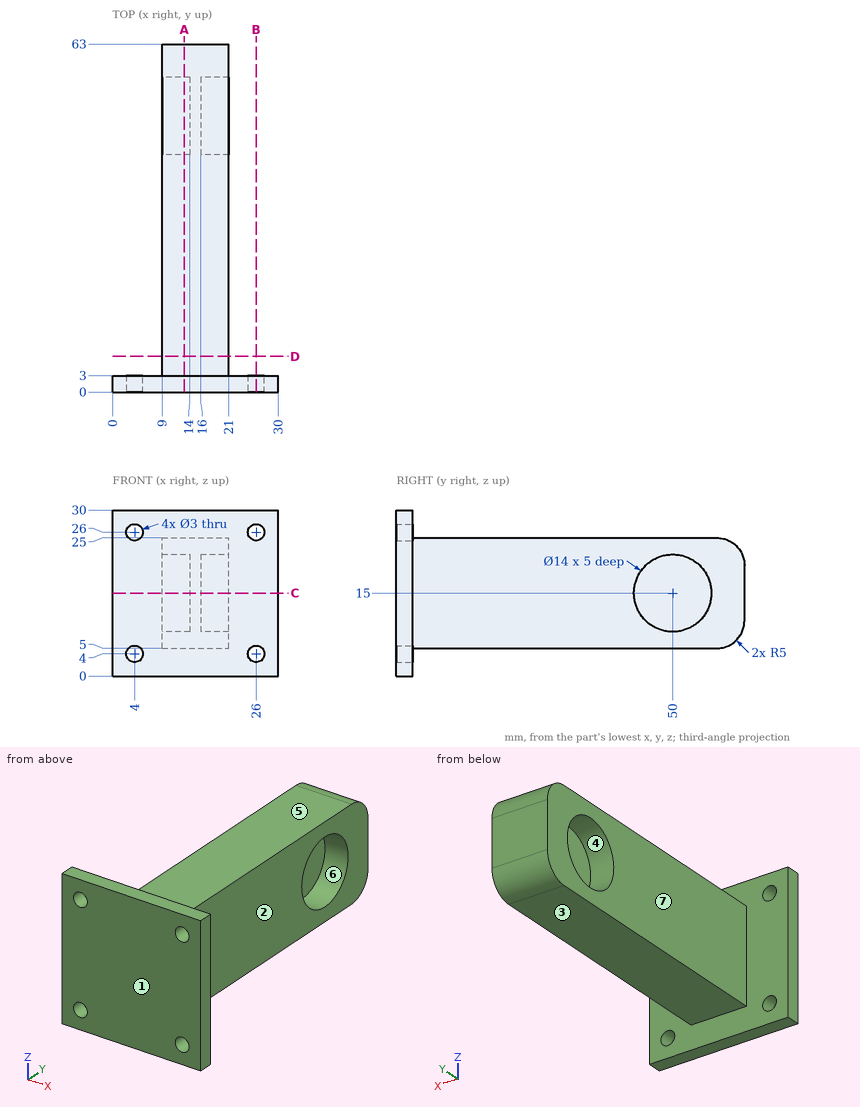
Job drawing, mm, ordinate dimensions from the low corner. One solid piece. A direction names the side the tool comes from. Give positions to 0.01 mm unless a question says otherwise; leave off trailing zeros. Write each loop counter-clockwise with the first axis right and the second up, starting at its lowest first coordinate (ties: lowest second). Pieces come first, ordered by that corner, then holes. Notation, with made-up numbers: (59, 70.25) - (92, 70.25) arc R22 cw to (92, 85.25) - close; hole circle Ø11 at (3.25, 75.25). An arc over 180 degrees is marked (long way). Answer as CSV lines item,"result".
1. Band-saw the part on C-C (z = 15). Write the cut outline in (x, y), and give its area (3 significant figures).
Responses:
outline,"(0, 0) - (30, 0) - (30, 3) - (21, 3) - (21, 43) - (16, 43) - (16, 57) - (21, 57) - (21, 63) - (9, 63) - (9, 57) - (14, 57) - (14, 43) - (9, 43) - (9, 3) - (0, 3) - close"
area,"670 mm2"
2. Pin check, flat tips, straight feed: pin 1 (18 mm diameter, centred on y = 50, z = 15, fed in from +X); pin 2 (3 mm diameter, centred on x = 19.5, y = 48.5, fed in from +Z); pin 3 (10 mm diameter, centred on y = 26, z = 14.5, fed in from -X); pin 4 (12 mm diameter, centred on x = 23, z = 13, fed in from +Y). Stop position of each tip, or through.
Responses:
pin 1,"stops at x = 21"
pin 2,"stops at z = 25"
pin 3,"stops at x = 9"
pin 4,"stops at y = 63"
3. Band-saw the part on A-A (x = 13). Write the cut outline in (y, z).
Responses:
outline,"(0, 0) - (3, 0) - (3, 5) - (58, 5) arc R5 ccw to (63, 10) - (63, 20) arc R5 ccw to (58, 25) - (3, 25) - (3, 30) - (0, 30) - close; hole circle Ø14 at (50, 15)"
4. Two-plate mould, pull along Z, no slides. Class the marked faces 4, 5, 6 and 7: +Z half, -Z half, draft (parallel to the pull), parting line (faces both ways), or undercut.
Responses:
face 4,"undercut"
face 5,"+Z half"
face 6,"undercut"
face 7,"draft"
5. 3-axis set-ups, long thin cutter, end or side, ignore diameter. For the marked faces 1, 2 and 3: which of +Z, -Z, +X, -X, +Y, -Y reach the whole face in a straight line?
Responses:
face 1,"+Z, -Z, +X, -X, -Y"
face 2,"+Z, -Z, +X, +Y"
face 3,"-Z, +X, -X, +Y"
6. Band-saw the part on D-D (y = 6.5). Write the cut outline in (x, z).
Responses:
outline,"(9, 5) - (21, 5) - (21, 25) - (9, 25) - close"
7. Band-saw the part on B-B (x = 26). Write the cut outline in (y, z).
Responses:
outline,"(0, 0) - (3, 0) - (3, 2.5) - (0, 2.5) - close; (0, 5.5) - (3, 5.5) - (3, 24.5) - (0, 24.5) - close; (0, 27.5) - (3, 27.5) - (3, 30) - (0, 30) - close"
8. Drill centre lines: L1, parallel to X at y = 30.5, z = 9; L2, parallel to Y at x = 23.5, z = 24.75; L3, parallel to Z at x = 13.75, y = 17.5. Where is each one in solid material? Low to high. Write a range as [from, to].
Responses:
L1,"x = [9, 21]"
L2,"y = [0, 3]"
L3,"z = [5, 25]"
